Part print with two shaded views. Sizes in mm from the minimum x, y, z corner. A direction names the side the tool comes from. Round coordinates to 2 decimals unless told otherwise and drop trailing zeros. Write each loop counter-clockwise with the first axis right and the second up, starting at its lowest first coordinate (ties: lowest second). Pieces come first, ordered by that corner, then holes. Notation, with made-up numbers: (-22, 0) - (-12, 0) arc R25 cw to (-12, 32) - close; hole circle Ø1 at (47.25, 63.5). An arc over 180 degrees is marked (long way). Use one line per item in the form item = value. Start each with the question number.
Item 1: Band-saw the part on A-A, the plane z = 1.25. List the corners of the cut face in (x, y).
Item 2: Band-saw the part on B-B, the plane x = 5. List the corners of the cut face in (y, z), and give its area (3 significant figures).
Item 3: Pin check, flat tips, straight feed: pin 1 (1 mm diameter, centred on x = 2, z = 7, fed in from +Y); pin 2 (3 mm diameter, centred on x = 5, y = 6, fed in from +Z); pin 3 (1 mm diameter, centred on y = 8.5, z = 5, fed in from -X). Stop position of each tip, or through.
Item 4: Band-saw the part on D-D, the plane x = 8.25. List the corners of the cut face in (y, z).
Item 5: Pull direction Y, two halves, no side cores. Call the marked faces 1, 2 and 3: +Y half, -Y half, draft (parallel to the pull), parting line (faces both ways), or undercut.
Item 6: Band-saw the part on C-C, the plane y = 6.75. List the corners of the cut face in (x, z).
Item 7: Tool access for the marked faces 4, 5 and 6: list every direction of +Z, -Z, +X, -X, +Y, -Y with a clear straight run to the whole face (end or side of a thin tool).
Item 8: Drill centre lines: L1, parallel to Y at x = 5, z = 5.5; L2, parallel to Z at x = 7.75, y = 1; L3, parallel to Y at x = 5, z = 2.25. Where is each one in solid material? Low to high.
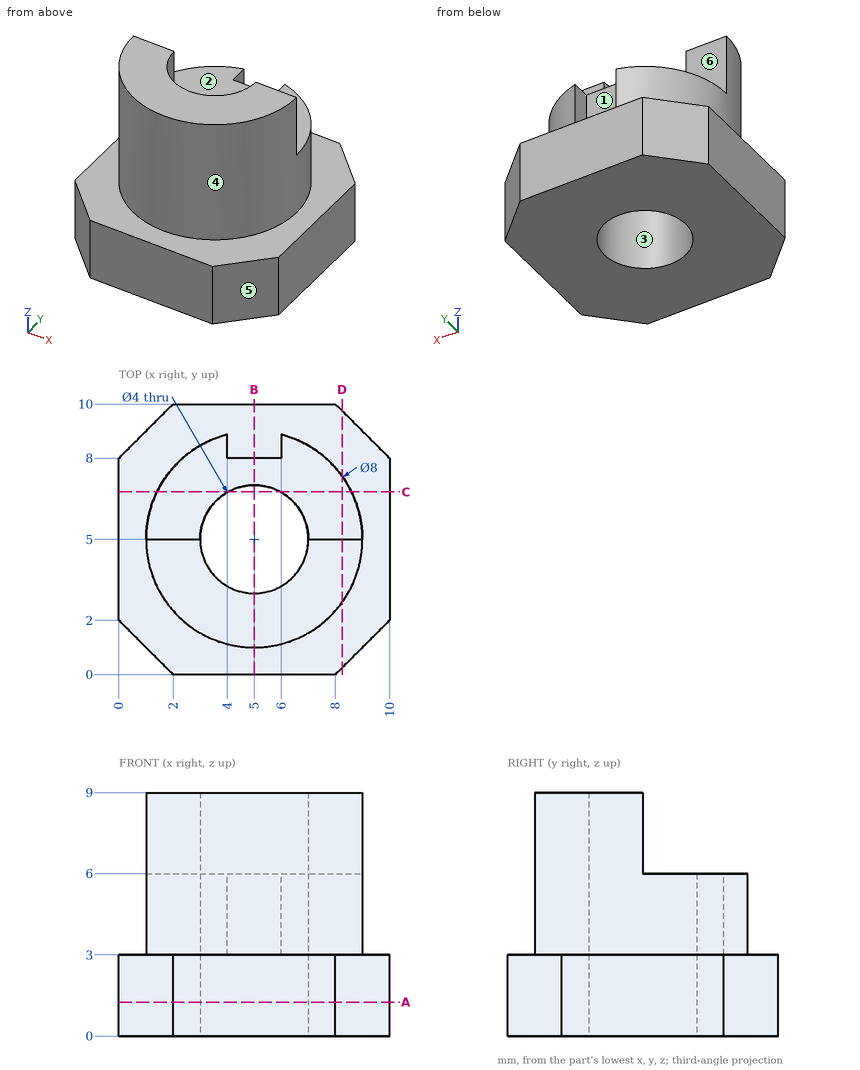
Determined:
q1.outline = (0, 2) - (2, 0) - (8, 0) - (10, 2) - (10, 8) - (8, 10) - (2, 10) - (0, 8) - close; hole circle Ø4 at (5, 5)
q2.outline = (0, 0) - (3, 0) - (3, 9) - (1, 9) - (1, 3) - (0, 3) - close; (7, 0) - (10, 0) - (10, 3) - (8, 3) - (8, 6) - (7, 6) - close
q2.area = 33.0 mm²
q3.pin_1 = 5
q3.pin_2 = 6
q3.pin_3 = 2.35
q4.outline = (0.25, 0) - (9.75, 0) - (9.75, 3) - (7.33, 3) - (7.33, 6) - (5, 6) - (5, 9) - (2.67, 9) - (2.67, 3) - (0.25, 3) - close
q5.face_1 = +Y half
q5.face_2 = draft
q5.face_3 = undercut
q6.outline = (0, 0) - (4.03, 0) - (4.03, 6) - (1.4, 6) - (1.4, 3) - (0, 3) - close; (5.97, 0) - (10, 0) - (10, 3) - (8.6, 3) - (8.6, 6) - (5.97, 6) - close
q7.face_4 = +Z
q7.face_5 = +Z, -Z, +X, -Y
q7.face_6 = +Z, +X, -X, +Y
q8.L1 = 1 to 3, 7 to 8
q8.L2 = 0 to 3
q8.L3 = 0 to 3, 7 to 10
